from build123d import *

# Parameters (mm, degrees)
SKETCH1_R           = 2
BOSS_EXTRUDE1_DEPTH = 2
FILLET1_R           = 4


with BuildPart() as part:
    # Sketch1 → Boss-Extrude1 (new body)
    with BuildSketch(Plane.XY):
        with BuildLine():
            Line((-36, 3.5), (-33, 3.5))
            ThreePointArc((-33, 3.5), (-16.705697773, 7.777052757), (0.096212134, 8.999054739))
            ThreePointArc((0.096212134, 8.999054739), (4.959049099, 3.369257867), (-1.158052235, -0.864282903))
            ThreePointArc((-1.158052235, -0.864282903), (-18.684835931, 0.519591906), (-35.800505276, -3.5))
            Line((-35.800505276, -3.5), (-50.800505276, -3.5))
            Line((-50.800505276, -3.5), (-50.800505276, 3.5))
            Line((-50.800505276, 3.5), (-36, 3.5))
        make_face()
        with Locations((-0.001007792, 4)):
            Circle(SKETCH1_R, mode=Mode.SUBTRACT)
        with Locations((-46.800505276, 0)):
            Circle(SKETCH1_R, mode=Mode.SUBTRACT)
        with Locations((-39.800505276, 0)):
            Circle(SKETCH1_R, mode=Mode.SUBTRACT)
    extrude(amount=BOSS_EXTRUDE1_DEPTH)

    # Fillet1
    fillet1_edges = [part.edges().sort_by_distance(p)[0] for p in [
        (-35.800505276, -3.5, 1),
        (-50.800505276, -3.5, 1),
    ]]
    fillet(fillet1_edges, radius=FILLET1_R)


solid = part.part
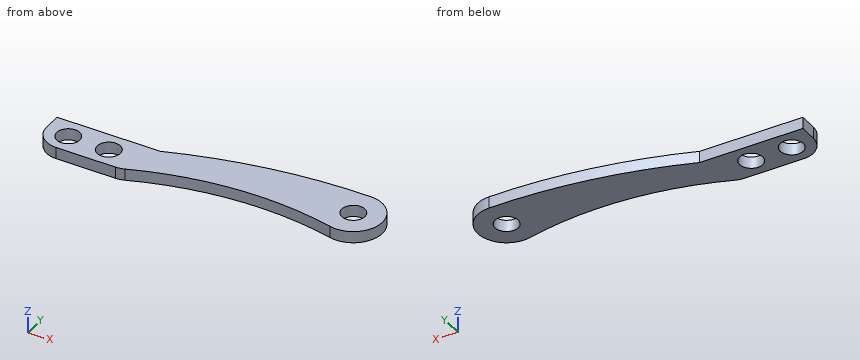
The listing builds one solid part. Answer for the finished solid, in the listing's coordinates (mm). Give positions to 0.01 mm unless a question says otherwise; leave off trailing zeros. Write each loop counter-clockwise with the first axis right and the second up, starting at its lowest first coordinate (ties: lowest second). Pieces come first, ordered by that corner, then holes.
Item 1: Find the intervals of material crossed by line 1 along Y through (x, z) = (-37.5, 0.3); line 2 along Y through (x, z) = (-46, 1.2); line 3 along X through (y, z) = (2.5, 1.25), in increasing order.
Item 2: Section C-C, the plane z = 0.3 is taken. Write down the section's boundary in (x, y), plus the area to 3 significant figures.
Item 3: Section B-B, the plane y = 0 is taken. Write down the section's boundary in (x, z), plus the area to 3 significant figures.
Item 4: A flat-ended cylindrical pin translates along its axis: P1, Ø0.6, axis at x = -43.5, z = 0.5, coming from the +Y side. Find the tip coordinate at first contact, or state that the pin passes through.
Item 5: Section A-A, the plane y = 4 is taken. Write down the section's boundary in (x, z).
Item 6: Section D-D, the plane y = 8 is taken. Write down the section's boundary in (x, z), plus the area to 3 significant figures.
Completed:
1. line 1: y = -3.5 to 3.5
1. line 2: y = -3.5 to -1.83, 1.83 to 3.5
1. line 3: x = -50.8 to -1.32, 1.32 to 4.77
2. outline: (-50.8, 0.5) arc R4 ccw to (-46.8, -3.5) - (-36.57, -3.5) arc R4 ccw to (-35.11, -3.23) arc R57.04 cw to (-1.16, -0.86) arc R5 ccw (long way) to (0.1, 9) arc R91.64 ccw to (-33, 3.5) - (-50.8, 3.5) - close; hole circle Ø4 at (-46.8, 0); hole circle Ø4 at (-39.8, 0); hole circle Ø4 at (0, 4)
2. area: 367 mm2
3. outline: (-50.77, 0) - (-48.8, 0) - (-48.8, 2) - (-50.77, 2) - close; (-44.8, 0) - (-41.8, 0) - (-41.8, 2) - (-44.8, 2) - close; (-37.8, 0) - (-23.16, 0) - (-23.16, 2) - (-37.8, 2) - close; (-5.55, 0) - (3, 0) - (3, 2) - (-5.55, 2) - close
3. area: 56.3 mm2
4. P1: stops at y = 3.5
5. outline: (-31.59, 0) - (-2, 0) - (-2, 2) - (-31.59, 2) - close; (2, 0) - (5, 0) - (5, 2) - (2, 2) - close
6. outline: (-15.3, 0) - (3, 0) - (3, 2) - (-15.3, 2) - close
6. area: 36.6 mm2
